from build123d import *

# Parameters (mm, degrees)
BOSS_EXTRUDE1_DEPTH = 18
SKETCH2_R           = 1.6
CUT_EXTRUDE1_DEPTH  = 32.827660926
FILLET1_R           = 3
CHAMFER1_SIZE       = 0.4


with BuildPart() as part:
    # Sketch1 → Boss-Extrude1 (new body)
    with BuildSketch(Plane.XY):
        with BuildLine():
            Line((-7.5, 0), (-5, 0))
            ThreePointArc((-5, 0), (0, 5), (5, 0))
            Line((5, 0), (7.5, 0))
            ThreePointArc((7.5, 0), (12.5, 5), (17.5, 0))
            Line((17.5, 0), (25, 0))
            Line((25, 0), (25, 8))
            Line((25, 8), (-25, 8))
            Line((-25, 8), (-25, 0))
            Line((-25, 0), (-17.5, 0))
            ThreePointArc((-17.5, 0), (-12.5, 5), (-7.5, 0))
        make_face()
    extrude(amount=BOSS_EXTRUDE1_DEPTH)

    # Sketch2 → Cut-Extrude1 (cut, through all)
    with BuildSketch(Plane(origin=(0, 8, 0), x_dir=(1, 0, 0), z_dir=(0, 1, 0))):
        with Locations(Location((-21, -9, 0), (0, 0, 270))):
            Circle(SKETCH2_R)
        with Locations(Location((21, -9, 0), (0, 0, 270))):
            Circle(SKETCH2_R)
    extrude(amount=-CUT_EXTRUDE1_DEPTH, mode=Mode.SUBTRACT)

    # Fillet1
    fillet1_edges = [part.edges().sort_by_distance(p)[0] for p in [
        (25, 4, 18),
        (-25, 4, 18),
    ]]
    fillet(fillet1_edges, radius=FILLET1_R)

    # Chamfer1
    chamfer1_edges = [part.edges().sort_by_distance(p)[0] for p in [
        (21, 8, 7.4),
        (-21, 8, 7.4),
        (12.5, 5, 0),
        (0, 5, 0),
        (-12.5, 5, 0),
        (0, 8, 0),
        (-25, 4, 0),
        (-25, 8, 7.5),
        (-24.121320344, 8, 17.121320344),
        (0, 8, 18),
        (24.121320344, 8, 17.121320344),
        (25, 8, 7.5),
        (25, 4, 0),
        (12.5, 5, 18),
        (0, 5, 18),
        (-12.5, 5, 18),
        (6.25, 0, 0),
        (-6.25, 0, 0),
        (6.25, 0, 18),
        (-6.25, 0, 18),
    ]]
    chamfer(chamfer1_edges, length=CHAMFER1_SIZE)


solid = part.part
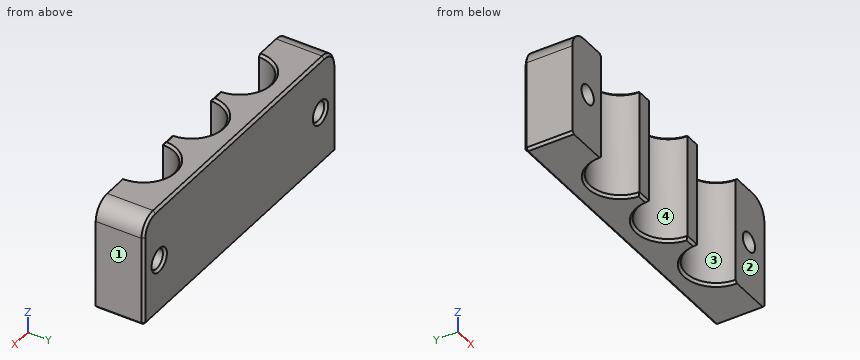
Read the model definition and answer for the solid it produces. Units are mm, in the model's axes. Face numbers are marked on the shaded views. Round coordinates to 2 decimals unless told otherwise and drop trailing zeros. Loops run counter-clockwise (first coordinate to the right, second up) from the corner with the lowest first, then second, coordinate; pieces in that order, holes last.
Q1. Each of these flat-tipped pins is pushed along its axis until it touches: pin 1 (3 mm diameter, centred on x = 3, z = 10.5, fed in from -Y); pin 2 (4 mm diameter, centred on x = 0.5, y = 2.5, fed in from +Z). Where does it stop, or does it pass through?
Q2. Section A-A on x = 21 is taken. Write down the section's boundary in (y, z), and give its area (3 significant figures).
Q3. Section D-D on z = 1.75 is taken. Write down the section's boundary in (x, y), and give its area (3 significant figures).
Q4. Section C-C on y = 6 is taken. Write down the section's boundary in (x, z), and give its area (3 significant figures).
Q5. Consider probe 1 along X at (y, z) = (5.25, 9); probe 2 along X at (y, z) = (3.25, 12); probe 3 along X at (y, z) = (4, 1.25). Determine where each line is inside the solid, lowest interval first.
Q6. Section B-B on z = 9 is taken. Write down the section's boundary in (x, y).
Q7. Determine the mould class of the marked faces 1, 2, 3 and 4 for opening direction X: released by +X, released by -X, zero draft, split by the parting line, or undercut.
Output:
1. pin 1: stops at y = 2.18
1. pin 2: passes through
2. outline: (0, 0) - (7.6, 0) - (8, 0.4) - (8, 7) - (7.6, 7.4) - (0, 7.4) - close; (0, 10.6) - (7.6, 10.6) - (8, 11) - (8, 17.6) - (7.6, 18) - (0, 18) - close
2. area: 118 mm2
3. outline: (-25, 0) - (-17.5, 0) arc R5 cw to (-7.5, 0) - (-5, 0) arc R5 cw to (5, 0) - (7.5, 0) arc R5 cw to (17.5, 0) - (25, 0) - (25, 7.6) - (24.6, 8) - (-24.6, 8) - (-25, 7.6) - close
3. area: 282 mm2
4. outline: (-25, 0.4) - (-24.6, 0) - (24.6, 0) - (25, 0.4) - (25, 15) arc R3 ccw to (22, 18) - (-22, 18) arc R3 ccw to (-25, 15) - close; hole circle Ø3.2 at (-21, 9); hole circle Ø3.2 at (21, 9)
4. area: 880 mm2
5. probe 1: x = -25 to -22.6, -19.4 to 19.4, 22.6 to 25
5. probe 2: x = -25 to -16.3, -8.7 to -3.8, 3.8 to 8.7, 16.3 to 25
5. probe 3: x = -25 to -15.5, -9.5 to -3, 3 to 9.5, 15.5 to 25
6. outline: (-25, 0) - (-22.6, 0) - (-22.6, 7.6) - (-23, 8) - (-24.6, 8) - (-25, 7.6) - close; (-19.4, 0) - (-17.5, 0) arc R5 cw to (-7.5, 0) - (-5, 0) arc R5 cw to (5, 0) - (7.5, 0) arc R5 cw to (17.5, 0) - (19.4, 0) - (19.4, 7.6) - (19, 8) - (-19, 8) - (-19.4, 7.6) - close; (22.6, 0) - (25, 0) - (25, 7.6) - (24.6, 8) - (23, 8) - (22.6, 7.6) - close
7. face 1: released by +X
7. face 2: zero draft
7. face 3: undercut
7. face 4: undercut
